from build123d import *

# Parameters (mm, degrees)
SKETCH1_W              = 101.6
SKETCH1_H              = 76.2
BOSS_EXTRUDE1_DEPTH    = 3.175
M3_5_CLEARANCE_HOLE1_D = 3.9
CUT_EXTRUDE6_DEPTH     = 64.816710194
CUT_EXTRUDE7_DEPTH     = 64.816710194
CIRPATTERN1_COUNT      = 4
CUT_EXTRUDE8_DEPTH     = 64.816710194


with BuildPart() as part:
    # Sketch1 → Boss-Extrude1 (new, symmetric)
    with BuildSketch(Plane(origin=(0, 0, 0), x_dir=(1, 0, 0), z_dir=(0, 1, 0))):
        Rectangle(SKETCH1_W, SKETCH1_H)
    extrude(amount=BOSS_EXTRUDE1_DEPTH, both=True)

    # M3.5 Clearance Hole1 (through all)
    with Locations(Plane(origin=(0, 3.175, 0), x_dir=(1, 0, 0), z_dir=(0, 1, 0))):
        with Locations((-15.5, 10.2), (15.5, 10.2), (15.5, -20.8), (-15.5, -20.8)):
            Hole(M3_5_CLEARANCE_HOLE1_D / 2)

    # Sketch23 → Cut-Extrude6 (cut, through all)
    with BuildSketch(Plane(origin=(0, 3.175, 0), x_dir=(1, 0, 0), z_dir=(0, 1, 0))):
        with BuildLine():
            Line((-12.9860741, 15.72), (-12.9860741, 11.800180167))
            ThreePointArc((-12.9860741, 11.800180167), (-13.392821792, 8.092821792), (-17.100180167, 7.6860741))
            Line((-17.100180167, 7.6860741), (-21.02, 7.6860741))
            Line((-21.02, 7.6860741), (-21.02, -18.2860741))
            Line((-21.02, -18.2860741), (-17.100180167, -18.2860741))
            ThreePointArc((-17.100180167, -18.2860741), (-13.392821792, -18.692821792), (-12.9860741, -22.400180167))
            Line((-12.9860741, -22.400180167), (-12.9860741, -26.32))
            Line((-12.9860741, -26.32), (12.9860741, -26.32))
            Line((12.9860741, -26.32), (12.9860741, -22.400180167))
            ThreePointArc((12.9860741, -22.400180167), (13.392821792, -18.692821792), (17.100180167, -18.2860741))
            Line((17.100180167, -18.2860741), (21.02, -18.2860741))
            Line((21.02, -18.2860741), (21.02, 7.6860741))
            Line((21.02, 7.6860741), (17.100180167, 7.6860741))
            ThreePointArc((17.100180167, 7.6860741), (13.392821792, 8.092821792), (12.9860741, 11.800180167))
            Line((12.9860741, 11.800180167), (12.9860741, 15.72))
            Line((12.9860741, 15.72), (-12.9860741, 15.72))
        make_face()
    extrude(amount=-CUT_EXTRUDE6_DEPTH, mode=Mode.SUBTRACT)

    # Sketch24 → Cut-Extrude7 (cut, through all)
    with BuildSketch(Plane(origin=(0, 3.175, 0), x_dir=(1, 0, 0), z_dir=(0, 1, 0))):
        with BuildLine():
            Line((-18.979586404, 8.233476566), (-19.479586404, 8.233476566))
            ThreePointArc((-19.479586404, 8.233476566), (-21.954460139, 7.2083503), (-22.979586404, 4.733476566))
            Line((-22.979586404, 4.733476566), (-22.979586404, -15.333476566))
            ThreePointArc((-22.979586404, -15.333476566), (-21.954460139, -17.8083503), (-19.479586404, -18.833476566))
            Line((-19.479586404, -18.833476566), (-18.979586404, -18.833476566))
            ThreePointArc((-18.979586404, -18.833476566), (-18.000834998, -18.693840487), (-17.100180167, -18.2860741))
            ThreePointArc((-17.100180167, -18.2860741), (-13.392821792, -18.692821792), (-12.9860741, -22.400180167))
            Line((-12.9860741, -22.400180167), (-7.9860741, -22.400180167))
            Line((-7.9860741, -22.400180167), (-7.9860741, 11.800180167))
            Line((-7.9860741, 11.800180167), (-12.9860741, 11.800180167))
            ThreePointArc((-12.9860741, 11.800180167), (-13.392821792, 8.092821792), (-17.100180167, 7.6860741))
            ThreePointArc((-17.100180167, 7.6860741), (-18.000834998, 8.093840487), (-18.979586404, 8.233476566))
        make_face()
    cut_extrude7 = extrude(amount=-CUT_EXTRUDE7_DEPTH, mode=Mode.SUBTRACT)

    # CirPattern1: Cut-Extrude7 ×4 about axis
    cirpattern1_axis = Axis((0, 0, 5.3), (0, 1, 0))
    for i in range(1, CIRPATTERN1_COUNT):
        add(cut_extrude7.rotate(cirpattern1_axis, i * 360 / CIRPATTERN1_COUNT), mode=Mode.SUBTRACT)

    # Sketch25 → Cut-Extrude8 (cut, through all)
    with BuildSketch(Plane(origin=(0, 3.175, 0), x_dir=(1, 0, 0), z_dir=(0, 1, 0))):
        with BuildLine():
            Line((-43.942, 28.194), (-43.942, 15.494))
            ThreePointArc((-43.942, 15.494), (-40.767, 12.319), (-37.592, 15.494))
            Line((-37.592, 15.494), (-37.592, 28.194))
            ThreePointArc((-37.592, 28.194), (-40.767, 31.369), (-43.942, 28.194))
        make_face()
        with BuildLine():
            Line((-43.942, -9.906), (-43.942, -22.606))
            ThreePointArc((-43.942, -22.606), (-40.767, -25.781), (-37.592, -22.606))
            Line((-37.592, -22.606), (-37.592, -9.906))
            ThreePointArc((-37.592, -9.906), (-40.767, -6.731), (-43.942, -9.906))
        make_face()
    cut_extrude8 = extrude(amount=-CUT_EXTRUDE8_DEPTH, mode=Mode.SUBTRACT)

    # Mirror1: Cut-Extrude8 across plane
    add(cut_extrude8.mirror(Plane(origin=(0, 0, 0), x_dir=(0, 0, 1), z_dir=(1, 0, 0))), mode=Mode.SUBTRACT)


solid = part.part
Design review of the part built by this model. Coordinates are the model's own, in mm. Give positions to 0.01 mm unless a question says otherwise; leave off trailing zeros. Write each loop counter-clockwise with the first axis right and the second up, starting at its lowest first coordinate (ties: lowest second). Pieces come first, ordered by that corner, then holes. Notation, with made-up numbers: M 66.25,63 L 122.25,63 A20 cw 122.25,98 Z; hole C 61,49 d11. An arc over 180 degrees is marked long. Return JSON: item names as keys, results as strings. Group by question number.
Item 1: Take a section at C-C (x = 15.5). Give the boundary of the cut face in (y, z) (3 decimals), plus the area to 3 significant figures.
Item 2: Take a section at A-A (x = 0). Give the boundary of the cut face in (y, z) (3 decimals).
Item 3: Clearance check with a flat-ended pin moving along its axis: pin 1 Ø3 at (x, z) = (15.5, 20.8) entering from -Y. State where the tip first meets the part, or that it passes through.
Item 4: Take a section at D-D (z = 20.8). Give the boundary of the cut face in (x, y) (3 decimals), plus the area to 3 significant figures.
Item 5: The part is to be moulded in two halves that separate along X. For faces 1 (the cylindrical face through (-12.48, 0.04, -16.68)), 2 (the flat face through (-50.8, 0, 1)), 3 (the cylindrical face through (-13.552, -0.044, -10.286)), say which applies: pulls with the +X half, pulls with the -X half, needs draft (parallel to the pull), parting line crosses it, or undercut.
Item 6: Wall thickness on line 1 along X through (y, z) = (2.25, 13); line 2 along Z through (x, y) = (15.5, -1); line 3 along X through (y, z) = (1.75, -10.2): over which ranges is each line inside the solid? List them lowest first.
Item 7: Take a section at B-B (z = -10.2). Give the boundary of the cut face in (x, y) (3 decimals), plus the area to 3 significant figures.
Return value:
{
 "1": {"outline": "M -3.175,-38.1 L 3.175,-38.1 L 3.175,-12.15 L -3.175,-12.15 Z; M -3.175,-8.25 L 3.175,-8.25 L 3.175,-7.22 L -3.175,-7.22 Z; M -3.175,17.82 L 3.175,17.82 L 3.175,18.85 L -3.175,18.85 Z; M -3.175,22.75 L 3.175,22.75 L 3.175,38.1 L -3.175,38.1 Z", "area": "275 mm2"},
 "2": {"outline": "M -3.175,-38.1 L 3.175,-38.1 L 3.175,-17.68 L -3.175,-17.68 Z; M -3.175,28.28 L 3.175,28.28 L 3.175,38.1 L -3.175,38.1 Z"},
 "3": {"pin 1": "passes through"},
 "4": {"outline": "M -50.8,-3.175 L -43.942,-3.175 L -43.942,3.175 L -50.8,3.175 Z; M -37.592,-3.175 L -17.45,-3.175 L -17.45,3.175 L -37.592,3.175 Z; M -13.55,-3.175 L -12.52,-3.175 L -12.52,3.175 L -13.55,3.175 Z; M 12.52,-3.175 L 13.55,-3.175 L 13.55,3.175 L 12.52,3.175 Z; M 17.45,-3.175 L 37.592,-3.175 L 37.592,3.175 L 17.45,3.175 Z; M 43.942,-3.175 L 50.8,-3.175 L 50.8,3.175 L 43.942,3.175 Z", "area": "356 mm2"},
 "5": {"face 1": "undercut", "face 2": "pulls with the -X half", "face 3": "undercut"},
 "6": {"line 1": "x = -50.8 to -43.94, -37.59 to -22.98, 22.98 to 37.59, 43.94 to 50.8", "line 2": "z = -38.1 to -12.15, -8.25 to -7.22, 17.82 to 18.85, 22.75 to 38.1", "line 3": "x = -50.8 to -17.45, -13.55 to -12.52, 12.52 to 13.55, 17.45 to 50.8"},
 "7": {"outline": "M -50.8,-3.175 L -17.45,-3.175 L -17.45,3.175 L -50.8,3.175 Z; M -13.55,-3.175 L -12.52,-3.175 L -12.52,3.175 L -13.55,3.175 Z; M 12.52,-3.175 L 13.55,-3.175 L 13.55,3.175 L 12.52,3.175 Z; M 17.45,-3.175 L 50.8,-3.175 L 50.8,3.175 L 17.45,3.175 Z", "area": "437 mm2"}
}
